from build123d import *

# Parameters (mm, degrees)
SKETCH1_W           = 82.55
SKETCH1_H           = 44.45
BOSS_EXTRUDE1_DEPTH = 6.35
SKETCH2_W           = 5.588
SKETCH2_H           = 18.288
BOSS_EXTRUDE2_DEPTH = 6.35
SKETCH5_W           = 18.288
SKETCH5_H           = 5.588
BOSS_EXTRUDE3_DEPTH = 6.35
SKETCH3_W           = 5.588
SKETCH3_H           = 18.288
CUT_EXTRUDE1_DEPTH  = 97.739994025
SKETCH6_R           = 1.524
CUT_EXTRUDE2_DEPTH  = 97.739994025


with BuildPart() as part:
    # Sketch1 → Boss-Extrude1 (new body)
    with BuildSketch(Plane.XY):
        with Locations((41.275, 22.225)):
            Rectangle(SKETCH1_W, SKETCH1_H)
    extrude(amount=BOSS_EXTRUDE1_DEPTH)

    # Sketch2 → Boss-Extrude2 (add)
    with BuildSketch(Plane.XY.offset(6.35)):
        with Locations((-2.794, 22.225)):
            Rectangle(SKETCH2_W, SKETCH2_H)
    extrude(amount=-BOSS_EXTRUDE2_DEPTH)

    # Sketch5 → Boss-Extrude3 (add)
    with BuildSketch(Plane.XY.offset(6.35)):
        with Locations((38.481, 47.244)):
            Rectangle(SKETCH5_W, SKETCH5_H)
        with Locations((38.481, -2.794)):
            Rectangle(SKETCH5_W, SKETCH5_H)
    extrude(amount=-BOSS_EXTRUDE3_DEPTH)

    # Sketch3 → Cut-Extrude1 (cut, through all)
    with BuildSketch(Plane.XY.offset(6.35)):
        with Locations((79.756, 22.225)):
            Rectangle(SKETCH3_W, SKETCH3_H)
    extrude(amount=-CUT_EXTRUDE1_DEPTH, mode=Mode.SUBTRACT)

    # Sketch6 → Cut-Extrude2 (cut, through all)
    with BuildSketch(Plane.XY.offset(6.35)):
        with Locations((-2.794, 22.225)):
            Circle(SKETCH6_R)
        with Locations((38.481, -2.794)):
            Circle(SKETCH6_R)
        with Locations((38.481, 47.244)):
            Circle(SKETCH6_R)
        Polygon((67.437, 23.8125), (70.612, 23.8125), (70.612, 26.035), (73.787, 26.035), (73.787, 23.8125), (76.962, 23.8125), (76.962, 20.6375), (73.787, 20.6375), (73.787, 18.415), (70.612, 18.415), (70.612, 20.6375), (67.437, 20.6375), align=None)
    extrude(amount=-CUT_EXTRUDE2_DEPTH, mode=Mode.SUBTRACT)


solid = part.part
Verification items for the finished model (mm, model axes). A direction names the side the tool comes from. Round coordinates to 2 decimals unless told otherwise and drop trailing zeros. Loops run counter-clockwise (first coordinate to the right, second up) from the corner with the lowest first, then second, coordinate; pieces in that order, holes last. Notation, with made-up numbers: M 2,29 L 19,29 A4 cw 19,34 Z; hole C 31.25,-40 d5. An arc over 180 degrees is marked long. Write each question's results on one line, items separated by ' | '.
1) Section check B-B on y = 39. Record the boundary of the cut face in (x, z), then the cut area to 3 significant figures.
Checks:
outline: M 0,0 L 82.55,0 L 82.55,6.35 L 0,6.35 Z | area: 524 mm2
2) Gauge pin test, flat ends, axial feed: P1, Ø1.9, axis at y = 39.5, z = 3, coming from the -X side; P2, Ø1.8, axis at x = 38.481, y = 47.244, coming from the +Z side; P3, Ø3, axis at x = -3, z = 2.5, coming from the +Y side; P4, Ø1.6, axis at x = 75, z = 3, coming from the -Y side. Record the tip position at first contact, or that the pin passes through.
Checks:
P1: stops at x = 0 | P2: passes through | P3: stops at y = 31.37 | P4: stops at y = 0
3) Scan lines: L1, parallel to X at y = 24.5, z = 2; L2, parallel to Y at x = 73, z = 0.75 (3 decimals); L3, parallel to Y at x = 53, z = 5.25. Record each from-to range of solid material in increasing order. Write a range as from..to.
Checks:
L1: x = -5.59..70.61, 73.79..76.96 | L2: y = 0..18.415, 26.035..44.45 | L3: y = 0..44.45
4) Section check C-C on z = 5.25. State how many separate pieces and enclosed holes the cut face has, then the cut area to 3 significant figures.
Checks:
separate pieces: 1 | enclosed holes: 3 | area: 3,810 mm2
5) Access from +Z, -Z, +X, -X, +Y, -Y to the whole of each face (thin tool, end or side, straight path). Record for faces 4 (the flat face through (47.625, 47, 3)), 5 (the flat face through (65, 0, 3)), 6 (the flat face through (67.437, 22, 3)).
Checks:
face 4: +Z, -Z, +X, +Y | face 5: +Z, -Z, +X, -Y | face 6: +Z, -Z, +X
6) Section check A-A on x = 66.5. Record the boundary of the cut face in (y, z), then the cut area to 3 significant figures.
Checks:
outline: M 0,0 L 44.45,0 L 44.45,6.35 L 0,6.35 Z | area: 282 mm2
7) Mould release check, pull along X, two halves, no side actions. Record for faces 1 (the flat face through (14, 0, 3)), 2 (the flat face through (0, 38, 3)), 3 (the cylindrical face through (39.889, -3.378, 3.219)): released by +X, released by -X, zero draft, split by the parting line, or undercut.
Checks:
face 1: zero draft | face 2: released by -X | face 3: undercut
